Source: CAD feature listing. Evaluate the final solid. Frame: model axes, mm. A direction names the side the tool comes from. Coordinates: 2 decimals unless noted, no trailing zeros. Write each loop counter-clockwise with the first axis right and the second up, starting at its lowest first coordinate (ties: lowest second). Pieces come first, ordered by that corner, then holes. Notation, with made-up numbers: (-30, 16.25) - (29, 16.25) arc R29 ccw to (29, 48.25) - close; hole circle Ø7 at (31, 86.25). An arc over 180 degrees is marked (long way). One line per item, written item: value.
Autodesk Inventor part; units mm, degrees
ref_plane "YZ Plane" through (0, 0, 0) normal (1, 0, 0) x (0, 1, 0)
ref_plane "XZ Plane" through (0, 0, 0) normal (0, 1, 0) x (-1, 0, 0)
ref_plane "XY Plane" through (0, 0, 0) normal (0, 0, 1) x (1, 0, 0)
sketch "Sketch1" plane through (0, 0, 0) normal (0, 1, 0) x (-1, 0, 0)
  line L0 (0, 0) -> (0, -152)
  line L1 (0, -152) -> (66, -152)
  line L2 (66, -152) -> (66, 0)
  line L3 (66, 0) -> (0, 0)
  line L4 (66, 0) -> (66, 3)
  line L5 (66, 3) -> (0, 3)
  line L6 (0, 3) -> (0, 0)
  line L7 (66, -152) -> (66, -155)
  line L8 (66, -155) -> (0, -155)
  line L9 (0, -155) -> (0, -152)
  line L10 (66, -155) -> (70, -155)
  line L11 (70, -155) -> (70, 3)
  line L12 (70, 3) -> (66, 3)
  dimension "d0" = 152
  dimension "d1" = 66
  dimension "d2" = 3
  dimension "d3" = 3
  dimension "d4" = 4
extrude "Extrusion1" add sketch "Sketch1" against normal blind 4
extrude "Extrusion2" add sketch "Sketch1" along normal blind 94 contours L4 L12 L11 L10 L7 L2
sketch "Sketch7" plane through (0, 0, 0) normal (0, 1, 0) x (1, 0, 0)
  line L0 (0, 155) -> (0, -3)
  line L1 (0, -3) -> (3, -3)
  line L2 (3, -3) -> (3, 155)
  line L3 (3, 155) -> (0, 155)
  line L4 (0, 155) -> (0, -3)
  point P0 (0, 0)
  dimension "d15" = 3
extrude "Extrusion3" add sketch "Sketch7" against normal up to surface (4 mm away)
extrude "Extrusion4" add sketch "Sketch7" along normal blind 15
sketch "Sketch8" plane through (-66, 94, -155) normal (0, 0, -1) x (-1, 0, 0)
  line L0 (-66, -79) -> (0, 0)
  line L1 (0, -94) -> (0, 0)
  line L2 (0, 0) -> (0, -94)
  line L3 (-66, -94) -> (0, -94)
  line L4 (0, -94) -> (-66, -94)
  line L5 (-66, -94) -> (-66, -79)
extrude "Extrusion5" add sketch "Sketch8" against normal blind 3
sketch "Sketch9" plane through (-70, 94, 3) normal (0, 0, 1) x (1, 0, 0)
  line L0 (0, 0) -> (4, 0)
  line L1 (70, -94) -> (70, -79)
  line L2 (4, 0) -> (70, -79)
  line L3 (70, -79) -> (70, -94)
  line L4 (4, -94) -> (70, -94)
  line L5 (70, -94) -> (4, -94)
  line L6 (4, -94) -> (4, 0)
  line L7 (4, -94) -> (4, 0)
extrude "Extrusion6" add sketch "Sketch9" against normal blind 3
sketch "Sketch10" plane through (0, 0, 0) normal (0, 1, 0) x (1, 0, 0)
  line L0 (-66, 0) -> (-66, 152)
  line L1 (-66, 0) -> (-66, 20)
  line L2 (-66, 20) -> (-51, 20)
  line L3 (-66, 0) -> (0, 0)
  line L4 (0, 0) -> (0, 20)
  line L5 (0, 152) -> (0, 0)
  line L6 (0, 20) -> (-15, 20)
  line L7 (0, 152) -> (0, 132)
  line L8 (0, 132) -> (-15, 132)
  line L9 (0, 152) -> (-66, 152)
  line L10 (-66, 152) -> (-66, 132)
  line L11 (-66, 132) -> (-51, 132)
  line L12 (-51, 132) -> (-51, 20)
  line L13 (-15, 20) -> (-51, 20)
  line L14 (-15, 20) -> (-15, 132)
  line L15 (-51, 132) -> (-15, 132)
  dimension "d24" = 20
  dimension "d25" = 15
  dimension "d26" = 20
  dimension "d27" = 15
  dimension "d28" = 20
  dimension "d29" = 20
  dimension "d30" = 15
extrude "Extrusion7" cut sketch "Sketch10" against normal up to surface (4 mm away) contours L12 L15 L14 L13
sketch "Sketch11" plane through (-66, 0, -152) normal (1, 0, 0) x (0, 0, -1)
  line L0 (-152, 94) -> (0, 94)
  line L1 (-152, 94) -> (-132, 94)
  line L2 (-132, 94) -> (-132, 79)
  line L3 (0, 94) -> (-20, 94)
  line L4 (-20, 94) -> (-20, 79)
  line L5 (-20, 79) -> (-132, 79)
  line L6 (0, 0) -> (-152, 0)
  line L7 (-152, 0) -> (-132, 0)
  line L8 (-132, 0) -> (-132, 15)
  line L9 (-132, 15) -> (-132, 79)
  line L10 (0, 0) -> (-20, 0)
  line L11 (-20, 0) -> (-20, 15)
  line L12 (-20, 15) -> (-20, 79)
  line L13 (-20, 15) -> (-132, 15)
  dimension "d33" = 20
  dimension "d34" = 15
  dimension "d35" = 20
  dimension "d36" = 15
  dimension "d37" = 20
  dimension "d38" = 15
  dimension "d39" = 20
  dimension "d40" = 15
extrude "Extrusion8" cut sketch "Sketch11" against normal up to surface (4 mm away) contours L5 L12 L13 L9
sketch "Sketch12" plane through (0, 0, 0) normal (0, 1, 0) x (1, 0, 0)
  line L0 (-70, -3) -> (3, -3)
  line L1 (3, -3) -> (3, 20)
  line L2 (3, -3) -> (3, 155)
  line L3 (3, -3) -> (3, 8.5)
  line L4 (3, 8.5) -> (-70, 8.5)
  line L5 (3, 8.5) -> (-17, 8.5)
  line L6 (-70, 8.5) -> (-50, 8.5)
  circle A0 centre (-17, 8.5) radius 2
  circle A1 centre (-50, 8.5) radius 2
  line L7 (-70, 155) -> (3, 155)
  line L8 (3, 155) -> (3, 143.5)
  line L9 (3, 143.5) -> (-70, 143.5)
  line L10 (-70, 155) -> (-70, -3)
  line L11 (3, 143.5) -> (-17, 143.5)
  line L12 (-70, 143.5) -> (-50, 143.5)
  circle A2 centre (-17, 143.5) radius 2
  circle A3 centre (-50, 143.5) radius 2
  dimension "d43" = 23
  dimension "d44" = 11.5
  dimension "d45" = 20
  dimension "d46" = 20
  dimension "d47" = 4
  dimension "d48" = 4
  dimension "d49" = 11.5
  dimension "d50" = 20
  dimension "d51" = 20
  dimension "d52" = 4
  dimension "d53" = 4
extrude "Extrusion9" cut sketch "Sketch12" against normal up to surface (4 mm away) contours A1 L4 | L4 A1 | A0 L4 | L4 A0 | A3 L9 | L9 A3 | A2 L9 | L9 A2
sketch "Sketch13" plane through (-66, 0, -152) normal (1, 0, 0) x (0, 0, -1)
  circle A0 centre (-143.0001, 84.1472) radius 1.4502
  circle A1 centre (-142.9999, 54.147) radius 1.4501
  circle A2 centre (-9, 84.1467) radius 1.4497
  circle A3 centre (-9.0001, 54.147) radius 1.4501
  point P0 (-152, 0)
extrude "Extrusion10" cut sketch "Sketch13" against normal up to surface (4 mm away)
sketch "Sketch14" plane through (-66, 0, -152) normal (1, 0, 0) x (0, 0, -1)
  circle A0 centre (-9, 84.1467) radius 1.4497
  line L0 (-9, 84.1467) -> (-9, 64.0437)
  circle A1 centre (-9, 64.0437) radius 4.767
  circle A2 centre (-143.0001, 84.1472) radius 1.4502
  line L1 (-143.0001, 84.1472) -> (-143.0001, 64.0437)
  circle A3 centre (-143.0001, 64.0437) radius 4.767
  point P0 (-152, 0)
  dimension "d58" = 20.103
  dimension "d59" = 9.534
extrude "Extrusion11" cut sketch "Sketch14" against normal up to surface (4 mm away) contours A1 | A3
sketch "Sketch15" plane through (0, 0, 0) normal (0, 1, 0) x (1, 0, 0)
  circle A0 centre (-50, 8.5) radius 2
  circle A1 centre (-50, 8.5) radius 4.5
  circle A2 centre (-17, 8.5) radius 2
  circle A3 centre (-17, 8.5) radius 4.5
  circle A4 centre (-50, 143.5) radius 2
  circle A5 centre (-50, 143.5) radius 4.5
  circle A6 centre (-17, 143.5) radius 2
  circle A7 centre (-17, 143.5) radius 4.5
  point P0 (0, 0)
  dimension "d68" = 9
  dimension "d69" = 9
  dimension "d70" = 9
  dimension "d71" = 9
extrude "Extrusion12" cut sketch "Sketch15" against normal blind 2
sketch "Sketch16" plane through (-66, 0, -152) normal (1, 0, 0) x (0, 0, -1)
  circle A0 centre (-143.0001, 84.1472) radius 1.4502
  circle A1 centre (-143.0001, 84.1472) radius 3
  circle A2 centre (-142.9999, 54.147) radius 1.4501
  circle A3 centre (-142.9999, 54.147) radius 3
  circle A4 centre (-9, 84.1467) radius 1.4497
  circle A5 centre (-9, 84.1467) radius 3
  circle A6 centre (-9.0001, 54.147) radius 1.4501
  circle A7 centre (-9.0001, 54.147) radius 3
  point P0 (-152, 0)
  dimension "d74" = 6
  dimension "d75" = 6
  dimension "d76" = 6
  dimension "d77" = 6
extrude "Extrusion13" cut sketch "Sketch16" against normal blind 2
properties part number "battery_box"
1) Draft query along Y for faces 6 (the flat face through (-33.5, 55.1, 1.5)), 7 (the flat face through (-33, -2, -132)), 8 (the cylindrical face through (-66.99, 56.68, -10.61)). Return one class per face: released by +Y, released by -Y, zero draft, split by the parting line, or undercut.
Values found:
face 6: released by +Y
face 7: zero draft
face 8: undercut
2) Reachability of faces 1 (the cylindrical face through (-17.98, -0.99, -139.11)), 2 (the flat face through (-68, 79, -77)), 3 (the flat face through (-68, 56, -10)), 4 (the cylindrical face through (-18.474, -2.986, -9.852)), 5 (the flat face through (1, 15, -77)) from +Z, -Z, +X, -X, +Y, -Y: full face, straight path, thin tool, end or side. Return the list, or none.
Values found:
face 1: +Y
face 2: +X, -X
face 3: +X
face 4: +Y, -Y
face 5: +Z, -Z, +X, +Y
3) Section query D-D on y = 77. Output: boundary loops of the cut face in (x, z), then the cut area to 3 significant figures.
Values found:
outline: (-70, -155) - (-51.8, -155) - (-51.8, -152) - (-66, -152) - (-66, -132) - (-70, -132) - close; (-70, -20) - (-66, -20) - (-66, 0) - (-51.8, 0) - (-51.8, 3) - (-70, 3) - close
area: 269 mm2
4) Contact query for flat-ended pins moving along their axis: P1, Ø8, axis at y = 64, z = -20.5, coming from the +X side; P2, Ø7, axis at x = -17, z = -143.5, coming from the +Y side; P3, Ø10, axis at x = -10.5, z = -60.5, coming from the +Y side. Output: stop coordinate, or through.
Values found:
P1: x = -66
P2: y = -2
P3: y = 0
5) Section query A-A on y = 10. Output: boundary loops of the cut face in (x, z), then the cut area to 3 significant figures.
Values found:
outline: (-70, -155) - (3, -155) - (3, 3) - (-70, 3) - close; hole (-66, -152) - (0, -152) - (0, 0) - (-66, 0) - close
area: 1,500 mm2
6) Section query B-B on z = -77.5. Output: boundary loops of the cut face in (x, y), then the cut area to 3 significant figures.
Values found:
outline: (-70, -4) - (-51, -4) - (-51, 0) - (-66, 0) - (-66, 15) - (-70, 15) - close; (-70, 79) - (-66, 79) - (-66, 94) - (-70, 94) - close; (-15, -4) - (3, -4) - (3, 15) - (0, 15) - (0, 0) - (-15, 0) - close
area: 313 mm2
7) Material intervals for line 1 (X direction, y = -3.3, z = -8.5); line 2 (X direction, y = -1, z = -8.5); line 3 (Z direction, x = -17, y = -1.45), sorted ascending.
Values found:
line 1: -70 to -52, -48 to -19, -15 to 3
line 2: -70 to -54.5, -45.5 to -21.5, -12.5 to 3
line 3: -155 to -148, -139 to -132, -20 to -13, -4 to 3
8) Section query C-C on x = -39.5. Output: boundary loops of the cut face in (y, z), then the cut area to 3 significant figures.
Values found:
outline: (-4, -155) - (62.28, -155) - (62.28, -152) - (0, -152) - (0, -132) - (-4, -132) - close; (-4, -20) - (0, -20) - (0, 0) - (62.28, 0) - (62.28, 3) - (-4, 3) - close
area: 558 mm2
